Here's how the part is built. I have some questions about the finished solid (model axes, mm). A direction names the side the tool comes from. Give positions to 0.01 mm unless a question says otherwise; leave off trailing zeros. Write each loop counter-clockwise with the first axis right and the second up, starting at its lowest first coordinate (ties: lowest second). Pieces come first, ordered by that corner, then holes. Notation, with made-up numbers: (62.25, 62) - (121.25, 62) arc R23 ccw to (121.25, 88) - close; hole circle Ø9 at (83.5, 0). An arc over 180 degrees is marked (long way). Use a Markdown table: item, result.
```python
from build123d import *

# Parameters (mm, degrees)
BASE_EXTRUDE_DEPTH  = 13.75
CUT_EXTRUDE1_DEPTH  = 7
BOSS_EXTRUDE1_DEPTH = 5
BOSS_EXTRUDE2_START = -25
BOSS_EXTRUDE2_DEPTH = 25
HOLE1_START         = -13.75
HOLE1_OUTLINE_R     = 5
HOLE1_DEPTH         = 27.5
LPATTERN1_COUNT     = 2
LPATTERN1_PITCH     = 72
FILLET1_R           = 5
FILLET2_R           = 5
FILLET3_R           = 2
FILLET4_R           = 2


# Read off the part's stored shape, not the designer's step: Hole1
with BuildPart() as part:
    # Sketch3 → Base-Extrude (new, symmetric)
    with BuildSketch(Plane.XY):
        with BuildLine():
            Line((0, 12.5), (27.5, 12.5))
            Line((27.5, 12.5), (27.5, -12.5))
            Line((27.5, -12.5), (0, -12.5))
            ThreePointArc((0, -12.5), (-12.5, 0), (0, 12.5))
        make_face()
    extrude(amount=BASE_EXTRUDE_DEPTH, both=True)

    # Sketch5 → Cut-Extrude1 (cut, symmetric)
    with BuildSketch(Plane.XY):
        with BuildLine():
            Line((20.75, 12.5), (20.75, -12.5))
            Line((20.75, -12.5), (0, -12.5))
            ThreePointArc((0, -12.5), (-12.5, 0), (0, 12.5))
            Line((0, 12.5), (20.75, 12.5))
        make_face()
    extrude(amount=CUT_EXTRUDE1_DEPTH, both=True, mode=Mode.SUBTRACT)

    # Sketch6 → Boss-Extrude1 (add, symmetric)
    with BuildSketch(Plane.XY):
        with BuildLine():
            Line((27.5, 12.5), (72, 12.5))
            ThreePointArc((72, 12.5), (84.5, 0), (72, -12.5))
            Line((72, -12.5), (27.5, -12.5))
            Line((27.5, -12.5), (27.5, 12.5))
        make_face()
    extrude(amount=BOSS_EXTRUDE1_DEPTH, both=True)

    # Sketch8 → Boss-Extrude2 (add)
    with BuildSketch(Plane(origin=(0, 12.5, 0), x_dir=(-1, 0, 0), z_dir=(0, 1, 0)).offset(BOSS_EXTRUDE2_START)):
        Polygon((-27.5, 13.75), (-27.5, 5), (-34.75, 5), align=None)
    boss_extrude2 = extrude(amount=BOSS_EXTRUDE2_DEPTH)

    # Mirror1: Boss-Extrude2 across plane
    add(boss_extrude2.mirror(Plane.XY))

    # Hole1 outline → Hole1 (cut)
    with BuildSketch(Plane.XY.offset(HOLE1_START)):
        Circle(HOLE1_OUTLINE_R)
    hole1 = extrude(amount=HOLE1_DEPTH, mode=Mode.SUBTRACT)

    # LPattern1: Hole1 ×2
    with Locations(*[(i * LPATTERN1_PITCH, 0, 0) for i in range(1, LPATTERN1_COUNT)]):
        add(hole1, mode=Mode.SUBTRACT)

    # Fillet1
    fillet1_edges = [part.edges().sort_by_distance(p)[0] for p in [
        (34.75, 0, 5),
        (34.75, 0, -5),
    ]]
    fillet(fillet1_edges, radius=FILLET1_R)

    # Fillet2
    fillet2_edges = [part.edges().sort_by_distance(p)[0] for p in [
        (27.5, 0, 13.75),
        (27.5, 0, -13.75),
    ]]
    fillet(fillet2_edges, radius=FILLET2_R)

    # Fillet3
    fillet3_edges = [part.edges().sort_by_distance(p)[0] for p in [
        (54.550233765, -12.5, 5),
        (84.5, 0, 5),
        (84.5, 0, -5),
        (54.550233765, -12.5, -5),
        (-12.5, 0, 13.75),
        (12.574766235, 12.5, -13.75),
        (-12.5, 0, -13.75),
        (12.574766235, 12.5, 13.75),
        (54.550233765, 12.5, 5),
        (54.550233765, 12.5, -5),
        (34.973315281, 12.5, 5.475044386),
        (34.973315281, -12.5, 5.475044386),
        (34.973315281, 12.5, -5.475044386),
        (34.973315281, -12.5, -5.475044386),
        (31.125, 12.5, -9.375),
        (31.125, -12.5, -9.375),
        (31.125, 12.5, 9.375),
        (27.276684719, 12.5, 13.274955614),
        (27.276684719, 12.5, -13.274955614),
        (12.574766235, -12.5, -13.75),
        (31.125, -12.5, 9.375),
        (12.574766235, -12.5, 13.75),
        (27.276684719, -12.5, 13.274955614),
        (27.276684719, -12.5, -13.274955614),
    ]]
    fillet(fillet3_edges, radius=FILLET3_R)

    # Fillet4
    fillet4_edges = [part.edges().sort_by_distance(p)[0] for p in [
        (20.75, 0, 7),
        (20.75, 0, -7),
    ]]
    fillet(fillet4_edges, radius=FILLET4_R)


solid = part.part
```
Item 1: If we section it at C-C, the plane x = 61: Write out the boundary of the cut face in (y, z).
Values:
| item | result |
|---|---|
| outline | (-12.5, -3) arc R2 ccw to (-10.5, -5) - (10.5, -5) arc R2 ccw to (12.5, -3) - (12.5, 3) arc R2 ccw to (10.5, 5) - (-10.5, 5) arc R2 ccw to (-12.5, 3) - close |
Item 2: If we section it at B-B, the plane z = -2: Write out the boundary of the cut face in (x, y), plus the area to 3 significant figures.
Values:
| item | result |
|---|---|
| outline | (20.75, -12.5) - (72, -12.5) arc R12.5 ccw to (72, 12.5) - (20.75, 12.5) - close; hole circle Ø10 at (72, 0) |
| area | 1,450 mm2 |
Item 3: For faces 1 (the cylindrical face through (54.31, -11.93, 4.4)), 2 (the cylindrical face through (54.31, -11.9, -4.43)), 3 (the flat face through (35, 12.5, 0)), which set-ups out of +Z, -Z, +X, -X, +Y, -Y let a thin tool reach every point of the face, with its end or its side?
Values:
| item | result |
|---|---|
| face 1 | +Z, +X, -Y |
| face 2 | -Z, +X, -Y |
| face 3 | +Z, -Z, +X, -X, +Y |
Item 4: If we section it at A-A, the plane y = 0: Count the separate pieces of the cut face and the enclosed holes in it, plus the area to 3 significant figures.
Values:
| item | result |
|---|---|
| separate pieces | 4 |
| enclosed holes | 0 |
| area | 1,030 mm2 |
Item 5: If we section it at D-D, the plane x = 1: Write out the boundary of the cut face in (y, z).
Values:
| item | result |
|---|---|
| outline | (-12.5, -11.75) arc R2 ccw to (-10.5, -13.75) - (-4.9, -13.75) - (-4.9, -7) - (-12.5, -7) - close; (-12.5, 7) - (-4.9, 7) - (-4.9, 13.75) - (-10.5, 13.75) arc R2 ccw to (-12.5, 11.75) - close; (4.9, -13.75) - (10.5, -13.75) arc R2 ccw to (12.5, -11.75) - (12.5, -7) - (4.9, -7) - close; (4.9, 7) - (12.5, 7) - (12.5, 11.75) arc R2 ccw to (10.5, 13.75) - (4.9, 13.75) - close |
Item 6: Thinking about a two-plate mould opening in Y: for faces 4 (the cylindrical face through (27.304, -0.147, -13.262)), 5 (the cylindrical face through (-1.08, -4.88, -10.42)), 6 (the cylindrical face through (54.79, 11.9, -4.43)), which applies, +Y half, -Y half, draft (parallel to the pull), parting line (faces both ways), or undercut?
Values:
| item | result |
|---|---|
| face 4 | draft |
| face 5 | undercut |
| face 6 | +Y half |
Item 7: Will these pins go through, and if not, where does the flat tip stop? pin 1 Ø1.5 at (y, z) = (-3.5, -7) entering from +X; pin 2 Ø3 at (y, z) = (-2.5, -1) entering from -X; pin 3 Ø7.5 at (x, y) = (-1.5, -0.5) entering from +Z; pin 4 Ø1.5 at (x, y) = (36.5, 2.5) entering from +Z.
Values:
| item | result |
|---|---|
| pin 1 | stops at x = 33.79 |
| pin 2 | stops at x = 20.75 |
| pin 3 | stops at z = 13.75 |
| pin 4 | stops at z = 5.19 |
Item 8: I need wall thicknesses on line 1 along Z through (x, y) = (11.5, 5.75); line 2 along Y through (x, z) = (0, 11); line 3 along X through (y, z) = (0, 0.5). Which ranges of each line are inside material? Lowest first, please. Write a range as [from, to].
Values:
| item | result |
|---|---|
| line 1 | z = [-13.75, -7], [7, 13.75] |
| line 2 | y = [-12.5, -5], [5, 12.5] |
| line 3 | x = [20.75, 67], [77, 84.5] |
